Autodesk Fusion 360 part; units mm, degrees
sketch "Sketch1" plane through (0, 0, 0) normal (0, 1, 0) x (1, 0, 0)
  line L0 (0, -25.4) -> (0, 0)
  line L1 (0, 0) -> (25.4, 0)
  line L2 (12.7, -12.7) -> (11.05, -11.05) construction
  line L3 (3.175, -25.4) -> (3.175, -3.175)
  line L4 (3.175, -3.175) -> (25.4, -3.175)
  line L5 (25.4, -3.175) -> (25.4, 0)
  line L6 (0, -25.4) -> (3.175, -25.4)
  dimension "d1" = 25.4
  dimension "d2" = 25.4
  dimension "d13" = 3.175
extrude "Extrude1" add sketch "Sketch1" along normal blind 168.2
hole "Hole3" at (3.175, 157.087, 14.2875) direction (-1, 0, 0) diameter 6.5 end through all
mirror "Mirror1" about plane through (0, 0, 0) normal (0, 1, 0) of bodies 1 merged
equation "d5 = ( 336.4 / 2 ) * 1 mm"
equation "d27 = ( 22.225 / 2 ) * 1 mm"
Part model, mm, in its own coordinate system. A direction names the side the tool comes from. Coordinates: 2 decimals unless noted, no trailing zeros. Order: outer loops, then holes, each group sorted by start corner. A loop starts at its lowest first (then second) coordinate and runs counter-clockwise, first axis right, second up. Notation, with made-up numbers: (59, 80) - (74, 80) arc R20 cw to (74, 85) - close; hole circle Ø7 at (39, 41.5). An arc over 180 degrees is marked (long way). Return JSON: item names as keys, results as strings. Group by question number.
Item 1: Cut at C-C (z = 21). List the corners of the cut face in (x, y) (3 decimals), plus the area to 3 significant figures.
Item 2: Pin check, flat tips, straight feed: pin 1 (4 mm diameter, centred on y = -157.09, z = 14.29, fed in from -X) (3 decimals); pin 2 (6 mm diameter, centred on x = 8.5, z = 4, fed in from +Y); pin 3 (10 mm diameter, centred on x = 22.5, y = 70, fed in from +Z) (3 decimals). Stop position of each tip, or through.
Item 3: Cut at B-B (y = -89). List the corners of the cut face in (x, z) (3 decimals).
Item 4: Cut at A-A (x = 21.5). List the corners of the cut face in (y, z) (3 decimals).
Item 5: Drill centre line: probe 1 along Z at (x, y) = (16, 51) (3 decimals). Where is it in solid material? Low to high. Write a range as from..to.
Item 6: Pull direction Z, two halves, no side cores. Call faces 1 (the face through (1.57, -160.31, 14.71)), 2 (the face through (14, -2, 3.175)), 3 (the face through (13, -2, 0)), 4 (the face through (2, 168.2, 7)): pulls with the +Z half, pulls with the -Z half, needs draft (parallel to the pull), parting line crosses it, or undercut.
Item 7: Which spindle directions (+Z, -Z, +X, -X, +Y, -Y) get a long thin tool onto all of the face, cutting with end or side? Do faces 5 (the face through (0, -2, 13)), 6 (the face through (3.175, -2, 14)). Say none if no direction does.
Check values:
{
 "1": {"outline": "(0, -168.2) - (3.175, -168.2) - (3.175, 168.2) - (0, 168.2) - close", "area": "1,070 mm2"},
 "2": {"pin 1": "passes through", "pin 2": "stops at y = 168.2", "pin 3": "stops at z = 3.175"},
 "3": {"outline": "(0, 0) - (25.4, 0) - (25.4, 3.175) - (3.175, 3.175) - (3.175, 25.4) - (0, 25.4) - close"},
 "4": {"outline": "(-168.2, 0) - (168.2, 0) - (168.2, 3.175) - (-168.2, 3.175) - close"},
 "5": {"probe 1": "z = 0..3.175"},
 "6": {"face 1": "undercut", "face 2": "pulls with the +Z half", "face 3": "pulls with the -Z half", "face 4": "needs draft"},
 "7": {"face 5": "+Z, -Z, -X, +Y, -Y", "face 6": "+Z, +X, +Y, -Y"}
}
